```python
from build123d import *

# Parameters (mm, degrees)
BOSS_EXTRUDE2_DEPTH      = 28
SKETCH3_W                = 18
SKETCH3_H                = 6.5
CUT_EXTRUDE9_DEPTH       = 19
CUT_EXTRUDE10_DEPTH      = 31.757112998
CUT_EXTRUDE10_DEPTH_BACK = 31.757112998
SKETCH4_R                = 2.5


with BuildPart() as part:
    # Sketch1 → Boss-Extrude2 (new body)
    with BuildSketch(Plane.XY):
        with BuildLine():
            Line((-4.358898944, 9), (4.358898944, 9))
            ThreePointArc((4.358898944, 9), (7.071067812, 7.071067812), (9, 4.358898944))
            Line((9, 4.358898944), (9, -4.358898944))
            ThreePointArc((9, -4.358898944), (7.071067812, -7.071067812), (4.358898944, -9))
            Line((4.358898944, -9), (-4.358898944, -9))
            ThreePointArc((-4.358898944, -9), (-7.071067812, -7.071067812), (-9, -4.358898944))
            Line((-9, -4.358898944), (-9, 4.358898944))
            ThreePointArc((-9, 4.358898944), (-7.071067812, 7.071067812), (-4.358898944, 9))
        make_face()
    extrude(amount=-BOSS_EXTRUDE2_DEPTH)

    # Sketch3 → Cut-Extrude9 (cut)
    with BuildSketch(Plane.XY):
        Rectangle(SKETCH3_W, SKETCH3_H)
    extrude(amount=-CUT_EXTRUDE9_DEPTH, mode=Mode.SUBTRACT)

    # Sketch4 → Cut-Extrude10 (cut, two sides: drawn at the far end of the back side and taken through both)
    with BuildSketch(Plane(origin=(0, 0, 0), x_dir=(1, 0, 0), z_dir=(0, 1, 0)).offset(-CUT_EXTRUDE10_DEPTH_BACK)):
        with Locations(Location((0, 8, 0), (0, 0, 270))):
            Circle(SKETCH4_R)
    extrude(amount=CUT_EXTRUDE10_DEPTH + CUT_EXTRUDE10_DEPTH_BACK, mode=Mode.SUBTRACT)


solid = part.part
```
Geometry: final body of the model. Coordinates: model frame, mm. A direction names the side the tool comes from. Give positions to 0.01 mm unless a question says otherwise; leave off trailing zeros. Loops run counter-clockwise (first coordinate to the right, second up) from the corner with the lowest first, then second, coordinate; pieces in that order, holes last. Notation, with made-up numbers: (-37, 22.5) -> (16, 22.5) arc R21 ccw to (16, 29.5) -> close; hole circle Ø11 at (20, 20). An arc over 180 degrees is marked (long way). Return JSON: item names as keys, results as strings.
Item 1: Mould query, pull axis X, two halves, no side actions, for faces 1 (the cylindrical face through (0.1, 6.1, -10.5)), 2 (the flat face through (0, 9, -14)), 3 (the cylindrical face through (7.1, -7.04, -13.8)), 4 (the cylindrical face through (0.1, -6.2, -10.5)). Classes: released by +X, released by -X, zero draft, split by the parting line, or undercut.
Filled in:
{"face 1": "undercut", "face 2": "zero draft", "face 3": "released by +X", "face 4": "undercut"}
Item 2: Section A-A, the plane x = 0. Output: boundary loops of the cut face in (y, z), plus the area to 3 significant figures.
Filled in:
{"outline": "(-9, -28) -> (9, -28) -> (9, -10.5) -> (3.25, -10.5) -> (3.25, -19) -> (-3.25, -19) -> (-3.25, -10.5) -> (-9, -10.5) -> close; (-9, -5.5) -> (-3.25, -5.5) -> (-3.25, 0) -> (-9, 0) -> close; (3.25, -5.5) -> (9, -5.5) -> (9, 0) -> (3.25, 0) -> close", "area": "323 mm^2"}
Item 3: Access query for faces 5 (the flat face through (0, 0, -19)), 6 (the flat face through (0, -6, 0)). Directions: +Z, -Z, +X, -X, +Y, -Y. A direction counts if a zero-diameter tool reaches every point of the face in a straight line with its end or side. Return the directions, or none.
Filled in:
{"face 5": "+Z, +X, -X", "face 6": "+Z, +X, -X, +Y, -Y"}
Item 4: Section D-D, the plane y = -7. Output: boundary loops of the cut face in (x, z).
Filled in:
{"outline": "(-7.14, -28) -> (7.14, -28) -> (7.14, 0) -> (-7.14, 0) -> close; hole circle Ø5 at (0, -8)"}
Item 5: Line query: line 1 (Y direction, x = -1.5, z = -11.5); line 2 (Z direction, x = 0, y = -4.7); line 3 (X direction, y = 6.05, z = -8). Output: solid intervals per line, ascending.
Filled in:
{"line 1": "-9 to -3.25, 3.25 to 9", "line 2": "-28 to -10.5, -5.5 to 0", "line 3": "-7.96 to -2.5, 2.5 to 7.96"}
Item 6: Pin query (flat end, axial travel): P1, Ø1.5, axis at y = 7, z = -8, coming from the -X side; P2, Ø1.5, axis at y = -5.5, z = -21.5, coming from the -X side. Return the tip coordinate at first contact, or that it passes through.
Filled in:
{"P1": "x = -7.81", "P2": "x = -8.8"}
Item 7: Section B-B, the plane z = -8. Output: boundary loops of the cut face in (x, y).
Filled in:
{"outline": "(-9, -4.36) arc R10 ccw to (-4.36, -9) -> (-2.5, -9) -> (-2.5, -3.25) -> (-9, -3.25) -> close; (-9, 3.25) -> (-2.5, 3.25) -> (-2.5, 9) -> (-4.36, 9) arc R10 ccw to (-9, 4.36) -> close; (2.5, -9) -> (4.36, -9) arc R10 ccw to (9, -4.36) -> (9, -3.25) -> (2.5, -3.25) -> close; (2.5, 3.25) -> (9, 3.25) -> (9, 4.36) arc R10 ccw to (4.36, 9) -> (2.5, 9) -> close"}
Item 8: Section C-C, the plane z = -17.5. Output: boundary loops of the cut face in (x, y).
Filled in:
{"outline": "(-9, -4.36) arc R10 ccw to (-4.36, -9) -> (4.36, -9) arc R10 ccw to (9, -4.36) -> (9, -3.25) -> (-9, -3.25) -> close; (-9, 3.25) -> (9, 3.25) -> (9, 4.36) arc R10 ccw to (4.36, 9) -> (-4.36, 9) arc R10 ccw to (-9, 4.36) -> close"}
